Autodesk Inventor part; units mm, degrees
ref_plane "YZ Plane" through (0, 0, 0) normal (1, 0, 0) x (0, 1, 0)
ref_plane "XZ Plane" through (0, 0, 0) normal (0, 1, 0) x (-1, 0, 0)
ref_plane "XY Plane" through (0, 0, 0) normal (0, 0, 1) x (1, 0, 0)
sketch "Sketch1" plane through (0, 0, 0) normal (0, 1, 0) x (-1, 0, 0)
  line L0 (0, 0) -> (-88.9, 0)
  line L1 (-88.9, 0) -> (-88.9, -12.7)
  line L2 (-88.9, -12.7) -> (0, -12.7)
  line L3 (0, -12.7) -> (0, 0)
  dimension "d0" = 88.9
  dimension "d1" = 12.7
extrude "Extrusion1" add sketch "Sketch1" along normal blind 2.54
fillet "Fillet1" radius 3.175 4 edges at (88.9, 1.27, 0) (88.9, 1.27, -12.7) (0, 1.27, -12.7) (0, 1.27, 0)
sketch "Sketch2" plane through (0, 2.54, 0) normal (0, 1, 0) x (1, 0, 0)
  line L0 (88.9, 3.175) -> (88.9, 9.525)
  line L1 (88.9, 6.35) -> (44.45, 6.35)
  circle A0 centre (44.45, 6.35) radius 4.445
  point P0 (0, 0)
  dimension "d5" = 44.45
  dimension "d6" = 8.89
extrude "Extrusion2" cut sketch "Sketch2" against normal blind 2.54
sketch "Sketch3" plane through (0, 2.54, 0) normal (0, 1, 0) x (1, 0, 0)
  line L0 (3.175, 0) -> (85.725, 0)
  line L1 (44.45, 0) -> (44.45, 12.7)
  line L2 (85.725, 12.7) -> (3.175, 12.7)
  line L3 (44.45, 6.35) -> (58.166, 6.35)
  point P0 (0, 0)
  dimension "d9" = 13.716
hole "Hole1" at (58.166, 2.54, -6.35) direction (0, -1, 0) diameter 2.794 end through all
sketch "Sketch4" plane through (0, 2.54, 0) normal (0, 1, 0) x (1, 0, 0)
  line L0 (85.725, 12.7) -> (3.175, 12.7)
  line L1 (44.45, 12.7) -> (44.45, 0)
  line L2 (3.175, 0) -> (85.725, 0)
  line L3 (44.45, 6.35) -> (30.734, 6.35)
  point P0 (0, 0)
  dimension "d17" = 13.716
hole "Hole2" at (30.734, 2.54, -6.35) direction (0, -1, 0) diameter 2.794 end through all
sketch "Sketch5" plane through (0, 2.54, 0) normal (0, 1, 0) x (1, 0, 0)
  line L0 (0, 9.525) -> (0, 3.175)
  line L1 (0, 6.35) -> (5.08, 6.35)
  point P0 (0, 0)
  dimension "d25" = 5.08
hole "Hole3" at (5.08, 2.54, -6.35) direction (0, -1, 0) diameter 2.794 end through all
sketch "Sketch6" plane through (0, 2.54, 0) normal (0, 1, 0) x (1, 0, 0)
  line L0 (88.9, 3.175) -> (88.9, 9.525)
  line L1 (88.9, 6.35) -> (83.82, 6.35)
  point P0 (0, 0)
  dimension "d33" = 5.08
hole "Hole4" at (83.82, 2.54, -6.35) direction (0, -1, 0) diameter 2.794 end through all
properties part number "Main Rod v1"
Design review of the part built by this model. Coordinates are the model's own, in mm. Coordinates: 2 decimals unless noted, no trailing zeros. Loops run counter-clockwise (first coordinate to the right, second up) from the corner with the lowest first, then second, coordinate; pieces in that order, holes last. Notation, with made-up numbers: (24, 0) - (72, 0) arc R30 cw to (72, 37) - close; hole circle Ø2 at (16.5, 45.5). An arc over 180 degrees is marked (long way). Use CSV: the item, a comma, the result in double quotes. Start each with the question number.
1) Consider section B-B on x = 83.82. Write out the cut boundary in (y, z).
2) Consider section D-D on x = 44.45. Write out the cut boundary in (y, z) (3 decimals), then the cut area to 3 significant figures.
3) The part is to be moulded in two halves that separate along X. For faces 1 (the cylindrical face through (87.95, 1.29, -0.91)), 2 (the cylindrical face through (4.136, 1.252, -7.38)), 3 (the flat face through (44, 1, 0)), say which applies: +X half, -X half, draft (parallel to the pull), parting line (faces both ways), or undercut.
4) Wall thickness on L1, parallel to X at y = 0.95, z = -6.35 (3 decimals); L2, parallel to Z at x = 83.82, y = 2; L3, parallel to X at y = 1.7, z = -6.75: over which ranges is each line inside the solid? List them lowest first. Write a range as from..to.
5) Consider section C-C on y = 0.65. Write out the cut boundary in (x, z) (3 decimals), then the cut area to 3 significant figures.
6) Consider section A-A on z = -6.35. Write out the cut boundary in (x, y) (3 decimals), then the cut area to 3 significant figures.
Geometry says:
1,outline,"(0, -12.7) - (2.54, -12.7) - (2.54, -7.75) - (0, -7.75) - close; (0, -4.95) - (2.54, -4.95) - (2.54, 0) - (0, 0) - close"
2,outline,"(0, -12.7) - (2.54, -12.7) - (2.54, -10.795) - (0, -10.795) - close; (0, -1.905) - (2.54, -1.905) - (2.54, 0) - (0, 0) - close"
2,area,"9.68 mm^2"
3,face 1,"+X half"
3,face 2,"undercut"
3,face 3,"draft"
4,L1,"0..3.683, 6.477..29.337, 32.131..40.005, 48.895..56.769, 59.563..82.423, 85.217..88.9"
4,L2,"-12.7..-7.75, -4.95..0"
4,L3,"0..3.74, 6.42..29.4, 32.07..40.02, 48.88..56.83, 59.5..82.48, 85.16..88.9"
5,outline,"(0, -9.525) arc R3.175 ccw to (3.175, -12.7) - (85.725, -12.7) arc R3.175 ccw to (88.9, -9.525) - (88.9, -3.175) arc R3.175 ccw to (85.725, 0) - (3.175, 0) arc R3.175 ccw to (0, -3.175) - close; hole circle Ø2.794 at (5.08, -6.35); hole circle Ø2.794 at (30.734, -6.35); hole circle Ø8.89 at (44.45, -6.35); hole circle Ø2.794 at (58.166, -6.35); hole circle Ø2.794 at (83.82, -6.35)"
5,area,"1,030 mm^2"
6,outline,"(0, 0) - (3.683, 0) - (3.683, 2.54) - (0, 2.54) - close; (6.477, 0) - (29.337, 0) - (29.337, 2.54) - (6.477, 2.54) - close; (32.131, 0) - (40.005, 0) - (40.005, 2.54) - (32.131, 2.54) - close; (48.895, 0) - (56.769, 0) - (56.769, 2.54) - (48.895, 2.54) - close; (59.563, 0) - (82.423, 0) - (82.423, 2.54) - (59.563, 2.54) - close; (85.217, 0) - (88.9, 0) - (88.9, 2.54) - (85.217, 2.54) - close"
6,area,"175 mm^2"
